Work out the finished part from the listing and answer in its coordinate system (mm). Give positions to 0.01 mm unless a question says otherwise; leave off trailing zeros. Order: outer loops, then holes, each group sorted by start corner. A loop starts at its lowest first (then second) coordinate and runs counter-clockwise, first axis right, second up. Notation, with made-up numbers: (78.5, 88.25) -> (87.5, 88.25) arc R21 cw to (87.5, 111.25) -> close; hole circle Ø1 at (-6.5, 52). An arc over 180 degrees is marked (long way). Answer as CSV lines item,"result". Start each with the question number.
1. A cutting plane is placed at D-D (y = 58). Give the vertices of the cut face in (x, z) (3 decimals).
2. A cutting plane is placed at A-A (y = 24). Give the vertices of the cut face in (x, z) (3 decimals).
3. A cutting plane is placed at C-C (x = 1.6). State how many separate pieces and enclosed holes the cut face has, then the cut area to 3 significant figures.
4. Find the intervals of material crossed by L1, parallel to Z at x = 0.4, y = 34; L2, parallel to Z at x = 1.25, y = 64; L3, parallel to Y at x = 1.2, z = 10 (3 decimals), in increasing order.
5. A cutting plane is placed at B-B (z = 180.5). Give the vertices of the cut face in (x, y) (3 decimals).
6. Flat-ended cylindrical pins translate along their axes: pin 1 (1 mm diameter, centred on x = 1, z = 33, fed in from +Y) (3 decimals); pin 2 (1 mm diameter, centred on x = 2, y = 1.5, fed in from +Z); pin 3 (1.5 mm diameter, centred on x = 1, z = 168, fed in from -Y) (3 decimals). Find the tip coordinate at first contact, or state that the pin passes through.
Autodesk Fusion 360 part; units mm, degrees
sketch "Sketch1" plane through (0, 0, 0) normal (1, 0, 0) x (0, 1, 0)
  line L0 (98.425, 139.7) -> (101.6, 139.7)
  line L1 (0, 101.6) -> (0, 114.3)
  line L2 (0, 127) -> (0, 139.7)
  line L3 (98.425, 114.3) -> (101.6, 114.3)
  line L4 (0, 127) -> (3.175, 127)
  line L5 (101.6, 101.6) -> (101.6, 88.9)
  line L6 (0, 101.6) -> (3.175, 101.6)
  line L7 (98.425, 0) -> (98.425, 203.2)
  line L8 (98.425, 114.3) -> (98.425, 101.6)
  line L9 (98.425, 88.9) -> (101.6, 88.9)
  line L10 (101.6, 0) -> (100.0125, 0)
  line L11 (98.425, 127) -> (101.6, 127)
  line L12 (98.425, 101.6) -> (101.6, 101.6)
  line L13 (98.425, 95.25) -> (98.425, 88.9)
  line L14 (3.175, 0) -> (3.175, 203.2)
  line L15 (101.6, 127) -> (101.6, 114.3)
  line L16 (3.175, 127) -> (3.175, 114.3)
  line L17 (3.175, 88.9) -> (0, 88.9)
  line L18 (98.425, 139.7) -> (98.425, 127)
  line L19 (3.175, 114.3) -> (0, 114.3)
  line L20 (3.175, 12.7) -> (3.175, 0)
  line L21 (3.175, 190.5) -> (3.175, 177.8)
  line L22 (3.175, 177.8) -> (0, 177.8)
  line L23 (101.6, 50.8) -> (101.6, 38.1)
  line L24 (3.175, 50.8) -> (3.175, 38.1)
  line L25 (98.425, 152.4) -> (101.6, 152.4)
  line L26 (98.425, 50.8) -> (101.6, 50.8)
  line L27 (98.425, 152.4) -> (98.425, 139.7)
  line L28 (3.175, 139.7) -> (0, 139.7)
  line L29 (0, 139.7) -> (0, 127)
  line L30 (3.175, 101.6) -> (3.175, 88.9)
  line L31 (98.425, 101.6) -> (98.425, 95.25)
  line L32 (98.425, 203.2) -> (98.425, 190.5)
  line L33 (101.6, 152.4) -> (101.6, 139.7)
  line L34 (101.6, 203.2) -> (101.6, 190.5)
  line L35 (3.175, 203.2) -> (3.175, 190.5)
  line L36 (0, 0) -> (11.0998, 0)
  line L37 (98.425, 177.8) -> (98.425, 165.1)
  line L38 (98.425, 127) -> (98.425, 114.3)
  line L39 (0, 165.1) -> (0, 152.4)
  line L40 (11.0998, 0) -> (6.0198, 0)
  line L41 (98.425, 88.9) -> (98.425, 76.2)
  line L42 (0, 38.1) -> (3.175, 38.1)
  line L43 (98.425, 38.1) -> (98.425, 25.4)
  line L44 (101.6, 177.8) -> (101.6, 165.1)
  line L45 (98.425, 12.7) -> (101.6, 12.7)
  line L46 (0, 177.8) -> (0, 190.5)
  line L47 (98.425, 177.8) -> (101.6, 177.8)
  line L48 (0, 76.2) -> (0, 88.9)
  line L49 (0, 114.3) -> (0, 101.6)
  line L50 (3.175, 190.5) -> (0, 190.5)
  line L51 (98.425, 190.5) -> (101.6, 190.5)
  line L52 (101.6, 0) -> (0, 0)
  line L53 (98.425, 38.1) -> (101.6, 38.1)
  line L54 (90.5002, 0) -> (95.5802, 0)
  line L55 (3.175, 203.2) -> (101.6, 203.2)
  line L56 (98.425, 76.2) -> (101.6, 76.2)
  line L57 (98.425, 165.1) -> (101.6, 165.1)
  line L58 (98.425, 63.5) -> (98.425, 50.8)
  line L59 (98.425, 25.4) -> (101.6, 25.4)
  line L60 (0, 0) -> (0, 12.7)
  line L61 (3.175, 63.5) -> (0, 63.5)
  line L62 (98.425, 63.5) -> (101.6, 63.5)
  line L63 (0, 152.4) -> (0, 165.1)
  line L64 (0, 152.4) -> (3.175, 152.4)
  line L65 (0, 25.4) -> (0, 38.1)
  line L66 (0, 0) -> (12.065, 0)
  line L67 (3.175, 50.8) -> (0, 50.8)
  line L68 (101.6, 203.2) -> (98.425, 203.2)
  line L69 (98.425, 190.5) -> (98.425, 177.8)
  line L70 (101.6, 76.2) -> (101.6, 63.5)
  line L71 (101.6, 0) -> (90.5002, 0)
  line L72 (3.175, 25.4) -> (3.175, 12.7)
  line L73 (98.425, 25.4) -> (98.425, 12.7)
  line L74 (3.175, 38.1) -> (3.175, 25.4)
  line L75 (0, 12.7) -> (3.175, 12.7)
  line L76 (0, 50.8) -> (0, 63.5)
  line L77 (0, 25.4) -> (3.175, 25.4)
  line L78 (3.175, 177.8) -> (3.175, 165.1)
  line L79 (101.6, 0) -> (98.425, 0)
  line L80 (101.6, 0) -> (85.725, 0)
  line L81 (101.6, 25.4) -> (101.6, 12.7)
  line L82 (3.175, 76.2) -> (0, 76.2)
  line L83 (98.425, 165.1) -> (98.425, 152.4)
  line L84 (3.175, 63.5) -> (3.175, 50.8)
  line L85 (3.175, 152.4) -> (3.175, 139.7)
  line L86 (98.425, 76.2) -> (98.425, 63.5)
  line L87 (3.175, 165.1) -> (0, 165.1)
  line L88 (98.425, 50.8) -> (98.425, 38.1)
  line L89 (3.175, 76.2) -> (3.175, 63.5)
  line L90 (0, 0) -> (3.175, 0)
  line L91 (3.175, 88.9) -> (3.175, 76.2)
  line L92 (98.425, 203.2) -> (98.425, 177.8)
  line L93 (3.175, 0) -> (3.175, 59.055)
  line L94 (7.62, 139.7) -> (51.5837, 114.2474)
  line L95 (49.9801, 111.4777) -> (6.0165, 136.9303)
  line L96 (6.0165, 136.9303) -> (7.62, 139.7)
  line L97 (93.7411, 193.04) -> (49.7434, 167.6463)
  line L98 (92.1413, 195.8119) -> (93.7411, 193.04)
  line L99 (48.1436, 170.4182) -> (92.1413, 195.8119)
  line L100 (3.175, 60.2676) -> (4.1957, 60.2676)
  line L101 (4.1957, 60.2676) -> (6.35, 60.2676)
  line L102 (6.35, 60.2676) -> (95.8689, 92.8088)
  line L103 (94.7755, 95.8167) -> (5.2566, 63.2754)
  line L104 (49.9801, 111.4777) -> (50.2, 111.3504)
  line L105 (50.2, 111.3504) -> (51.8035, 114.1201)
  line L106 (51.8035, 114.1201) -> (51.5837, 114.2474)
  line L107 (95.8689, 92.8088) -> (96.1076, 92.8956)
  line L108 (96.1076, 92.8956) -> (95.0142, 95.9034)
  line L109 (95.0142, 95.9034) -> (94.7755, 95.8167)
  line L110 (49.7434, 167.6463) -> (49.5234, 167.5194)
  line L111 (49.5234, 167.5194) -> (47.9236, 170.2912)
  line L112 (47.9236, 170.2912) -> (48.1436, 170.4182)
  line L113 (5.2566, 63.2754) -> (6.35, 60.2676)
  dimension "d9" = 11.0998
  dimension "d10" = 11.0998
  dimension "d14" = 5.08
  dimension "d15" = 5.08
  dimension "d27" = 3.175
  dimension "d28" = 3.175
  dimension "d40" = 3.175
  dimension "d41" = 3.175
  dimension "d42" = 12.7
  dimension "d43" = 12.7
  dimension "d44" = 12.7
  dimension "d45" = 12.7
  dimension "d46" = 12.7
  dimension "d47" = 12.7
  dimension "d48" = 12.7
  dimension "d49" = 12.7
  dimension "d50" = 6.35
  dimension "d51" = 6.35
  dimension "d52" = 12.7
  dimension "d53" = 12.7
  dimension "d54" = 12.7
  dimension "d55" = 12.7
  dimension "d56" = 12.7
  dimension "d57" = 12.7
  dimension "d74" = 59.055
  dimension "d78" = 50.8
  dimension "d79" = 3.2004
  dimension "d80" = 50.8
  dimension "d81" = 50.8
  dimension "d82" = 3.2004
  dimension "d83" = 50.8
  dimension "d84" = 95.25
  dimension "d85" = 3.2004
  dimension "d86" = 95.25
  dimension "d87" = 0.254
  dimension "d88" = 0.254
  dimension "d89" = 3.2004
  dimension "d90" = 0.254
  dimension "d91" = 3.2004
extrude "Extrude1" add sketch "Sketch1" along normal blind 3.175
sketch "Sketch2" plane through (0, 0, 0) normal (1, 0, 0) x (0, 1, 0)
equation "d9 = 0.5 in - 0.063 in"
Answer sheet:
1,outline,"(0, 0) -> (3.175, 0) -> (3.175, 79.043) -> (0, 79.043) -> close; (0, 82.448) -> (3.175, 82.448) -> (3.175, 172.412) -> (0, 172.412) -> close; (0, 176.107) -> (3.175, 176.107) -> (3.175, 203.2) -> (0, 203.2) -> close"
2,outline,"(0, 0) -> (3.175, 0) -> (3.175, 66.684) -> (0, 66.684) -> close; (0, 70.089) -> (3.175, 70.089) -> (3.175, 126.519) -> (0, 126.519) -> close; (0, 130.217) -> (3.175, 130.217) -> (3.175, 203.2) -> (0, 203.2) -> close"
3,separate pieces,"1"
3,enclosed holes,"3"
3,area,"19,400 mm^2"
4,L1,"z = 0 to 70.32, 73.72 to 120.73, 124.43 to 203.2"
4,L2,"z = 0 to 81.22, 84.63 to 175.87, 179.57 to 203.2"
4,L3,"y = 0 to 98.425"
5,outline,"(0, 0) -> (3.175, 0) -> (3.175, 65.612) -> (0, 65.612) -> close; (0, 72.014) -> (3.175, 72.014) -> (3.175, 98.425) -> (0, 98.425) -> close"
6,pin 1,"stops at y = 98.425"
6,pin 2,"stops at z = 190.5"
6,pin 3,"stops at y = 3.175"
